The model under review builds one solid part; all positions refer to its coordinate system, in mm. Give positions to 0.01 mm unless a question says otherwise; leave off trailing zeros. Loops run counter-clockwise (first coordinate to the right, second up) from the corner with the lowest first, then second, coordinate; pieces in that order, holes last. Notation, with made-up numbers: M -34,-1.75 L -4,-1.75 A29 ccw -4,31.25 Z; hole C 80.5,18 d11. An arc over 180 degrees is marked long. Put each result on its own line as item: value. Start each with the question number.
Autodesk Inventor part; units mm, degrees
ref_plane "YZ Plane" through (0, 0, 0) normal (1, 0, 0) x (0, 1, 0)
ref_plane "XZ Plane" through (0, 0, 0) normal (0, 1, 0) x (-1, 0, 0)
ref_plane "XY Plane" through (0, 0, 0) normal (0, 0, 1) x (1, 0, 0)
sketch "Sketch1" plane through (0, 0, 0) normal (0, 0, 1) x (1, 0, 0)
  line L0 (-112.3194, 91.5028) -> (-340.9194, 91.5028)
  line L1 (-340.9194, 91.5028) -> (-340.9194, 66.1028)
  line L2 (-340.9194, 66.1028) -> (-112.3194, 66.1028)
  line L3 (-112.3194, 66.1028) -> (-112.3194, 91.5028)
  point P0 (0, 0)
  dimension "d0" = 228.6
  dimension "d1" = 25.4
extrude "Extrusion1" add sketch "Sketch1" along normal blind 25.4
shell "Shell1" thickness 3.175 removed faces 2 at (-112.3194, 74.5695, 8.4667) at (-340.9194, 83.0362, 8.4667)
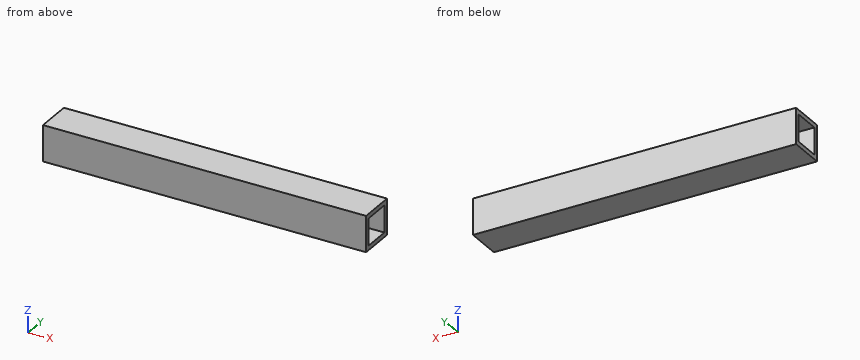
Item 1: Consider section B-B, the plane x = -243.5. Write out the cut boundary in (y, z) (3 decimals), plus the area to 3 significant figures.
Item 2: Consider section A-A, the plane y = 80.25. Write out the cut boundary in (x, z) (3 decimals).
Item 3: To check wall thickness, follow L1, parallel to Y at x = -238.5, z = 22; L2, parallel to Z at x = -136.5, y = 75 (3 decimals). State the ranges of each line that lie inside material, in increasing order. Write a range as [from, to].
Item 4: Consider section C-C, the plane z = 14.25. Write out the cut boundary in (x, y), plus the area to 3 significant figures.
Item 5: Clearance check with a flat-ended pin moving along its axis: pin 1 Ø5 at (y, z) = (87, 17) entering from +X. State where the tip first meets the part, or that it passes through.
Report:
1. outline: M 66.103,0 L 91.503,0 L 91.503,25.4 L 66.103,25.4 Z; hole M 69.278,3.175 L 88.328,3.175 L 88.328,22.225 L 69.278,22.225 Z
1. area: 282 mm²
2. outline: M -340.919,0 L -112.319,0 L -112.319,3.175 L -340.919,3.175 Z; M -340.919,22.225 L -112.319,22.225 L -112.319,25.4 L -340.919,25.4 Z
3. L1: [66.1, 69.28], [88.33, 91.5]
3. L2: [0, 3.175], [22.225, 25.4]
4. outline: M -340.92,66.1 L -112.32,66.1 L -112.32,69.28 L -340.92,69.28 Z; M -340.92,88.33 L -112.32,88.33 L -112.32,91.5 L -340.92,91.5 Z
4. area: 1,450 mm²
5. pin 1: x = -112.32
